```python
from build123d import *

# Parameters (mm, degrees)
CROQUIS1_R              = 0.25
SALIENTE_EXTRUIR1_DEPTH = 0.2
CROQUIS2_R              = 0.5
CROQUIS2_R_2            = 0.25
SALIENTE_EXTRUIR2_DEPTH = 0.2


with BuildPart() as part:
    # Croquis1 → Saliente-Extruir1 (new body)
    with BuildSketch(Plane.XY):
        with BuildLine():
            Line((-0.5, 7), (-0.25, 7))
            Line((-0.25, 7), (-0.5, 2.5))
            Line((-0.5, 2.5), (-0.25, 1.479019946))
            ThreePointArc((-0.25, 1.479019946), (0, -1.5), (0.25, 1.479019946))
            Line((0.25, 1.479019946), (0.5, 2.5))
            Line((0.5, 2.5), (0.25, 7))
            Line((0.25, 7), (0.5, 7))
            ThreePointArc((0.5, 7), (0.75, 7.25), (0.5, 7.5))
            Line((0.5, 7.5), (1.25, 9.5))
            Line((1.25, 9.5), (0.125, 12.5))
            Line((0.125, 12.5), (0.125, 17.5))
            Line((0.125, 17.5), (-0.125, 17.5))
            Line((-0.125, 17.5), (-0.125, 12.5))
            Line((-0.125, 12.5), (-1.25, 9.5))
            Line((-1.25, 9.5), (-0.5, 7.5))
            ThreePointArc((-0.5, 7.5), (-0.75, 7.25), (-0.5, 7))
        make_face()
        Circle(CROQUIS1_R, mode=Mode.SUBTRACT)
        Polygon((0, 7.5), (-1, 9.5), (0, 12.5), (1, 9.5), align=None, mode=Mode.SUBTRACT)
    extrude(amount=SALIENTE_EXTRUIR1_DEPTH)

    # Croquis2 → Saliente-Extruir2 (add)
    with BuildSketch(Plane(origin=(0, 0, 0), x_dir=(-1, 0, 0), z_dir=(0, 0, -1))):
        Circle(CROQUIS2_R)
        Circle(CROQUIS2_R_2, mode=Mode.SUBTRACT)
    extrude(amount=SALIENTE_EXTRUIR2_DEPTH)


solid = part.part
```
The listing builds one solid part. Answer for the finished solid, in the listing's coordinates (mm). Give positions to 0.01 mm unless a question says otherwise; leave off trailing zeros. Write each loop counter-clockwise with the first axis right and the second up, starting at its lowest first coordinate (ties: lowest second). Pieces come first, ordered by that corner, then holes. Notation, with made-up numbers: M -35.5,45 L 5.5,45 A24 ccw 5.5,58 Z; hole C -13,88 d1. An arc over 180 degrees is marked long. Write each question's results on one line, items separated by ' | '.
Q1. Section C-C, the plane y = 11 is taken. Write down the section's boundary in (x, z).
Output values:
outline: M -0.69,0 L -0.5,0 L -0.5,0.2 L -0.69,0.2 Z; M 0.5,0 L 0.69,0 L 0.69,0.2 L 0.5,0.2 Z
Q2. Section A-A, the plane y = 0 is taken. Write down the section's boundary in (x, z), then the cut area to 3 significant figures.
Output values:
outline: M -1.5,0 L -0.5,0 L -0.5,-0.2 L -0.25,-0.2 L -0.25,0.2 L -1.5,0.2 Z; M 0.25,-0.2 L 0.5,-0.2 L 0.5,0 L 1.5,0 L 1.5,0.2 L 0.25,0.2 Z | area: 0.600 mm2
Q3. Flat-ended cylindrical pins translate along their axes: P1, Ø1.5, axis at x = 0, y = 11, coming from the -Z side; P2, Ø1.5, axis at x = -0.5, y = 10.5, coming from the +Z side. Find the tip coordinate at first contact, or state that the pin passes through.
Output values:
P1: z = 0 | P2: z = 0.2
Q4. Section B-B, the plane z = 0.1 is taken. Write down the section's boundary in (x, y) (3 decimals), then the cut area to 3 significant figures.
Output values:
outline: M -1.25,9.5 L -0.5,7.5 A0.25 ccw -0.5,7 L -0.25,7 L -0.5,2.5 L -0.25,1.479 A1.5 ccw long 0.25,1.479 L 0.5,2.5 L 0.25,7 L 0.5,7 A0.25 ccw 0.5,7.5 L 1.25,9.5 L 0.125,12.5 L 0.125,17.5 L -0.125,17.5 L -0.125,12.5 Z; hole M -1,9.5 L 0,7.5 L 1,9.5 L 0,12.5 Z; hole C 0,0 d0.5 | area: 15.6 mm2
Q5. Section D-D, the plane y = 14 is taken. Write down the section's boundary in (x, z) (3 decimals).
Output values:
outline: M -0.125,0 L 0.125,0 L 0.125,0.2 L -0.125,0.2 Z
Q6. Consider L1, parallel to Y at x = 0, z = -0.1; L2, parallel to X at y = 0, z = 0.1; L3, parallel to Z at x = 1.2, y = 0.5. Determine where each line is inside the solid, lowest interval first. Write a range as from..to.
Output values:
L1: -0.5..-0.25, 0.25..0.5 | L2: -1.5..-0.25, 0.25..1.5 | L3: 0..0.2
